Part model, mm, in its own coordinate system. Coordinates: 2 decimals unless noted, no trailing zeros. Loops run counter-clockwise (first coordinate to the right, second up) from the corner with the lowest first, then second, coordinate; pieces in that order, holes last.
```python
from build123d import *

# Parameters (mm, degrees)
F0_R     = 59.53125
F0_R_2   = 46.83125
F0_R_3   = 34.13125
F1_DEPTH = 9.525
F3_DEPTH = 25.4


with BuildPart() as f1:
    # F0 (on Front) → F1 (new body)
    with BuildSketch(Plane.XZ):
        Circle(F0_R)
        Circle(F0_R_2, mode=Mode.SUBTRACT)
        Circle(F0_R_2)
        Circle(F0_R_3, mode=Mode.SUBTRACT)
    extrude(amount=F1_DEPTH)

    # F2 (on face) → F3 (cut)
    with BuildSketch(Plane.XZ.offset(9.525)):
        with BuildLine():
            Line((38.1, 0), (42.8625, 0))
            ThreePointArc((42.8625, 0), (40.48125, 2.38125), (38.1, 0))
        make_face()
        with BuildLine():
            ThreePointArc((38.1, 0), (40.48125, -2.38125), (42.8625, 0))
            Line((42.8625, 0), (38.1, 0))
        make_face()
        with BuildLine():
            ThreePointArc((55.5625, 0), (53.18125, 2.38125), (50.8, 0))
            Line((50.8, 0), (55.5625, 0))
        make_face()
        with BuildLine():
            Line((55.5625, 0), (50.8, 0))
            ThreePointArc((50.8, 0), (53.18125, -2.38125), (55.5625, 0))
        make_face()
        with BuildLine():
            ThreePointArc((0, -38.1), (-2.38125, -40.48125), (0, -42.8625))
            Line((0, -42.8625), (0, -38.1))
        make_face()
        with BuildLine():
            Line((0, -38.1), (0, -42.8625))
            ThreePointArc((0, -42.8625), (1.6837980227, -42.1650480227), (2.38125, -40.48125))
            ThreePointArc((2.38125, -40.48125), (1.6837980227, -38.7974519773), (0, -38.1))
        make_face()
        with BuildLine():
            Line((0, -55.5625), (0, -50.8))
            ThreePointArc((0, -50.8), (-2.38125, -53.18125), (0, -55.5625))
        make_face()
        with BuildLine():
            ThreePointArc((2.38125, -53.18125), (1.6837980227, -51.4974519773), (0, -50.8))
            Line((0, -50.8), (0, -55.5625))
            ThreePointArc((0, -55.5625), (1.6837980227, -54.8650480227), (2.38125, -53.18125))
        make_face()
        with BuildLine():
            ThreePointArc((-38.1, 0), (-40.48125, 2.38125), (-42.8625, 0))
            Line((-42.8625, 0), (-38.1, 0))
        make_face()
        with BuildLine():
            Line((-38.1, 0), (-42.8625, 0))
            ThreePointArc((-42.8625, 0), (-40.48125, -2.38125), (-38.1, 0))
        make_face()
        with BuildLine():
            Line((-55.5625, 0), (-50.8, 0))
            ThreePointArc((-50.8, 0), (-53.18125, 2.38125), (-55.5625, 0))
        make_face()
        with BuildLine():
            ThreePointArc((-55.5625, 0), (-53.18125, -2.38125), (-50.8, 0))
            Line((-50.8, 0), (-55.5625, 0))
        make_face()
        with BuildLine():
            ThreePointArc((0, 55.5625), (-2.38125, 53.18125), (0, 50.8))
            Line((0, 50.8), (0, 55.5625))
        make_face()
        with BuildLine():
            Line((0, 55.5625), (0, 50.8))
            ThreePointArc((0, 50.8), (1.6837980227, 51.4974519773), (2.38125, 53.18125))
            ThreePointArc((2.38125, 53.18125), (1.6837980227, 54.8650480227), (0, 55.5625))
        make_face()
        with BuildLine():
            ThreePointArc((2.38125, 40.48125), (1.6837980227, 42.1650480227), (0, 42.8625))
            Line((0, 42.8625), (0, 38.1))
            ThreePointArc((0, 38.1), (1.6837980227, 38.7974519773), (2.38125, 40.48125))
        make_face()
        with BuildLine():
            Line((0, 38.1), (0, 42.8625))
            ThreePointArc((0, 42.8625), (-2.38125, 40.48125), (0, 38.1))
        make_face()
    extrude(amount=-F3_DEPTH, mode=Mode.SUBTRACT)


solid = f1.part
```
Q1. Drop flat-ended pins along their axis: P1, Ø4.5, axis at x = -53.18, z = 0, coming from the -Y side; P2, Ø5, axis at y = -3.5, z = 19, coming from the -X side; P3, Ø5.5, axis at x = 53.18, z = 0, coming from the -Y side (3 decimals); P4, Ø4, axis at x = -17.5, y = -3.5, coming from the +Z side. Give the stop position or say it passes through.
Q2. Probe line 1 (Z direction, x = 0, y = -8.5); line 2 (X direction, y = -4.5, z = -52.5); line 3 (Z direction, x = -10, y = -4.25). List the from-to ranges inside material, lowest first.
Q3. Saw through at C-C (x = 0). List the corners of the cut face in (y, z) (1 decimal), plus the area to 3 significant figures.
Q4. Saw through at A-A (z = 0). List the corners of the cut face in (x, y) (1 decimal).
Q5. Mould opens along Z. For faces 1 (the flat face through (26, -9.525, -26)), 2 (the cylindrical face through (-47.242, -4.696, -36.224)), 3 (the cylindrical face through (-42.75, -4.83, -0.72)) say: released by +Z, released by -Z, zero draft, split by the parting line, or undercut.
Q6. Saw through at D-D (y = -6). Count the separate pieces of the cut face and the enclosed holes in it, plus the area to 3 significant figures.
Q7. Saw through at B-B (x = 23). List the corners of the cut face in (y, z) (3 decimals), plus the area to 3 significant figures.
Checked values:
1. P1: passes through
1. P2: stops at x = -57.2
1. P3: stops at y = -9.525
1. P4: stops at z = 57.48
2. line 1: z = -59.53 to -55.56, -50.8 to -42.86, -38.1 to -34.13, 34.13 to 38.1, 42.86 to 50.8, 55.56 to 59.53
2. line 2: x = -28.07 to -2.28, 2.28 to 28.07
2. line 3: z = -58.69 to -32.63, 32.63 to 58.69
3. outline: (-9.5, -59.5) - (0, -59.5) - (0, -55.6) - (-9.5, -55.6) - close; (-9.5, -50.8) - (0, -50.8) - (0, -42.9) - (-9.5, -42.9) - close; (-9.5, -38.1) - (0, -38.1) - (0, -34.1) - (-9.5, -34.1) - close; (-9.5, 34.1) - (0, 34.1) - (0, 38.1) - (-9.5, 38.1) - close; (-9.5, 42.9) - (0, 42.9) - (0, 50.8) - (-9.5, 50.8) - close; (-9.5, 55.6) - (0, 55.6) - (0, 59.5) - (-9.5, 59.5) - close
3. area: 302 mm2
4. outline: (-59.5, -9.5) - (-55.6, -9.5) - (-55.6, 0) - (-59.5, 0) - close; (-50.8, -9.5) - (-42.9, -9.5) - (-42.9, 0) - (-50.8, 0) - close; (-38.1, -9.5) - (-34.1, -9.5) - (-34.1, 0) - (-38.1, 0) - close; (34.1, -9.5) - (38.1, -9.5) - (38.1, 0) - (34.1, 0) - close; (42.9, -9.5) - (50.8, -9.5) - (50.8, 0) - (42.9, 0) - close; (55.6, -9.5) - (59.5, -9.5) - (59.5, 0) - (55.6, 0) - close
5. face 1: zero draft
5. face 2: split by the parting line
5. face 3: undercut
6. separate pieces: 1
6. enclosed holes: 9
6. area: 7,330 mm2
7. outline: (-9.525, -54.909) - (0, -54.909) - (0, -25.218) - (-9.525, -25.218) - close; (-9.525, 25.218) - (0, 25.218) - (0, 54.909) - (-9.525, 54.909) - close
7. area: 566 mm2
